from build123d import *

# Parameters (mm, degrees)
SKETCH_2_R               = 5
EXTRUDE_1_DEPTH          = 2.5
SKETCH_3_R               = 2.1
CUT_EXTRUDE_1_DEPTH      = 2.5
EXTRUDE_2_DEPTH          = 2.5
SKETCH_5_R               = 2.1
CUT_EXTRUDE_2_DEPTH      = 10
CUT_EXTRUDE_3_DEPTH      = 10
SKETCH_10_R              = 4
CUT_EXTRUDE_5_DEPTH      = 1
SKETCH_11_R              = 10
SKETCH_11_R_2            = 5
CUT_EXTRUDE_6_DEPTH      = 131.938989117
PATTERN_CIRCULAR_1_COUNT = 6


with BuildPart() as part:
    # 草图2 → 凸台-拉伸1 (new body)
    with BuildSketch(Plane(origin=(0, 0, 0), x_dir=(1, 0, 0), z_dir=(0, 1, 0))):
        Polygon((-54.5, 0), (-27.25, -47.198384506), (27.25, -47.198384506), (54.5, 0), (27.25, 47.198384506), (-27.25, 47.198384506), align=None)
        with Locations(Location((0, 0, 0), (0, 0, 270))):
            Circle(SKETCH_2_R, mode=Mode.SUBTRACT)
    extrude(amount=EXTRUDE_1_DEPTH)

    # 草图3 → 切除-拉伸1 (cut)
    with BuildSketch(Plane(origin=(0, 2.5, 0), x_dir=(1, 0, 0), z_dir=(0, 1, 0))):
        with Locations(Location((-22.5, 38.97114317, 0), (0, 0, 270))):
            Circle(SKETCH_3_R)
        with Locations(Location((22.5, 38.97114317, 0), (0, 0, 270))):
            Circle(SKETCH_3_R)
        with Locations(Location((45, 0, 0), (0, 0, 270))):
            Circle(SKETCH_3_R)
        with Locations(Location((22.5, -38.97114317, 0), (0, 0, 270))):
            Circle(SKETCH_3_R)
        with Locations(Location((-22.5, -38.97114317, 0), (0, 0, 270))):
            Circle(SKETCH_3_R)
        with Locations(Location((-45, 0, 0), (0, 0, 270))):
            Circle(SKETCH_3_R)
    extrude(amount=-CUT_EXTRUDE_1_DEPTH, mode=Mode.SUBTRACT)

    # 草图4 → 凸台-拉伸2 (add)
    with BuildSketch(Plane(origin=(0, 2.5, 0), x_dir=(1, 0, 0), z_dir=(0, 1, 0))):
        Polygon((-100.688021535, 0), (-50.344010768, -87.198384506), (50.344010768, -87.198384506), (100.688021535, 0), (50.344010768, 87.198384506), (-50.344010768, 87.198384506), align=None)
        Polygon((-54.5, 0), (-27.25, -47.198384506), (27.25, -47.198384506), (54.5, 0), (27.25, 47.198384506), (-27.25, 47.198384506), align=None, mode=Mode.SUBTRACT)
    extrude(amount=-EXTRUDE_2_DEPTH)

    # 草图5 → 切除-拉伸2 (cut)
    with BuildSketch(Plane(origin=(0, 2.5, 0), x_dir=(1, 0, 0), z_dir=(0, 1, 0))):
        with Locations(Location((-39, 67.549981495, 0), (0, 0, 270))):
            Circle(SKETCH_5_R)
        with Locations(Location((39, 67.549981495, 0), (0, 0, 270))):
            Circle(SKETCH_5_R)
        with Locations(Location((78, 0, 0), (0, 0, 270))):
            Circle(SKETCH_5_R)
        with Locations(Location((39, -67.549981495, 0), (0, 0, 270))):
            Circle(SKETCH_5_R)
        with Locations(Location((-39, -67.549981495, 0), (0, 0, 270))):
            Circle(SKETCH_5_R)
        with Locations(Location((-78, 0, 0), (0, 0, 270))):
            Circle(SKETCH_5_R)
    extrude(amount=-CUT_EXTRUDE_2_DEPTH, mode=Mode.SUBTRACT)

    # 草图8 → 切除-拉伸3 (cut)
    with BuildSketch(Plane(origin=(0, 2.5, 0), x_dir=(1, 0, 0), z_dir=(0, 1, 0))):
        with BuildLine():
            ThreePointArc((-38.999999879, 87.198384506), (-34.02771086, 86.55882369), (-29.37912053, 84.681777055))
            ThreePointArc((-29.37912053, 84.681777055), (2.23e-07, 76.996854011), (29.379120918, 84.681777273))
            ThreePointArc((29.379120918, 84.681777273), (34.027711134, 86.558823762), (39, 87.198384506))
            Line((39, 87.198384506), (-38.999999879, 87.198384506))
        make_face()
        with BuildLine():
            ThreePointArc((-58.647009902, 67.78395331), (-57.948284774, 72.748274003), (-56.016016118, 77.374183058))
            Line((-56.016016118, 77.374183058), (-95.016015856, 9.824202017))
            ThreePointArc((-95.016015856, 9.824202017), (-91.975995068, 13.810550415), (-88.026129369, 16.897824439))
            ThreePointArc((-88.026129369, 16.897824439), (-66.68123126, 38.498427568), (-58.647009902, 67.78395331))
        make_face()
        with BuildLine():
            ThreePointArc((-56.016016118, 77.374183058), (-48.824201425, 84.565997693), (-38.999999879, 87.198384506))
            Line((-38.999999879, 87.198384506), (-50.344010768, 87.198384506))
            Line((-50.344010768, 87.198384506), (-56.016016118, 77.374183058))
        make_face()
        with BuildLine():
            Line((50.344010768, 87.198384506), (39, 87.198384506))
            ThreePointArc((39, 87.198384506), (48.824200892, 84.565998001), (56.016015443, 77.374184228))
            Line((56.016015443, 77.374184228), (50.344010768, 87.198384506))
        make_face()
        with BuildLine():
            ThreePointArc((-95.016016282, -9.824201279), (-97.648403011, 4.26e-07), (-95.016015856, 9.824202017))
            Line((-95.016015856, 9.824202017), (-100.688021535, 0))
            Line((-100.688021535, 0), (-95.016016282, -9.824201279))
        make_face()
        with BuildLine():
            ThreePointArc((56.016015443, 77.374184228), (57.948284693, 72.7482743), (58.64700991, 67.783952574))
            ThreePointArc((58.64700991, 67.783952574), (66.681231635, 38.498426919), (88.026130025, 16.89782405))
            ThreePointArc((88.026130025, 16.89782405), (91.975995629, 13.810549846), (95.016016274, 9.824201294))
            Line((95.016016274, 9.824201294), (56.016015443, 77.374184228))
        make_face()
        with BuildLine():
            Line((-95.016016282, -9.824201279), (-56.016017948, -77.374179889))
            ThreePointArc((-56.016017948, -77.374179889), (-57.948285332, -72.748271969), (-58.647009908, -67.783952751))
            ThreePointArc((-58.647009908, -67.783952751), (-66.681232791, -38.498424916), (-88.026134156, -16.897821598))
            ThreePointArc((-88.026134156, -16.897821598), (-91.975997324, -13.810548132), (-95.016016282, -9.824201279))
        make_face()
        with BuildLine():
            Line((100.688021535, 0), (95.016016274, 9.824201294))
            ThreePointArc((95.016016274, 9.824201294), (97.648403011, -1.459e-06), (95.016014815, -9.824203821))
            Line((95.016014815, -9.824203821), (100.688021535, 0))
        make_face()
        with BuildLine():
            ThreePointArc((95.016014815, -9.824203821), (91.975994622, -13.810550865), (88.02613007, -16.897824023))
            ThreePointArc((88.02613007, -16.897824023), (66.681231717, -38.498426777), (58.647009914, -67.783952298))
            ThreePointArc((58.647009914, -67.783952298), (57.948284908, -72.748273515), (56.016016118, -77.374183058))
            Line((56.016016118, -77.374183058), (95.016014815, -9.824203821))
        make_face()
        with BuildLine():
            ThreePointArc((-39, -87.198384506), (-48.824203062, -84.565996748), (-56.016017948, -77.374179889))
            Line((-56.016017948, -77.374179889), (-50.344010768, -87.198384506))
            Line((-50.344010768, -87.198384506), (-39, -87.198384506))
        make_face()
        with BuildLine():
            Line((-39, -87.198384506), (39.000000014, -87.198384506))
            ThreePointArc((39.000000014, -87.198384506), (34.027710452, -86.558823583), (29.379119676, -84.681776576))
            ThreePointArc((29.379119676, -84.681776576), (-7.65e-07, -76.996854011), (-29.37912101, -84.681777325))
            ThreePointArc((-29.37912101, -84.681777325), (-34.027711185, -86.558823775), (-39, -87.198384506))
        make_face()
        with BuildLine():
            Line((50.344010768, -87.198384506), (56.016016118, -77.374183058))
            ThreePointArc((56.016016118, -77.374183058), (48.824201483, -84.565997659), (39.000000014, -87.198384506))
            Line((39.000000014, -87.198384506), (50.344010768, -87.198384506))
        make_face()
    extrude(amount=-CUT_EXTRUDE_3_DEPTH, mode=Mode.SUBTRACT)

    # 草图10 → 切除-拉伸5 (cut)
    with BuildSketch(Plane(origin=(0, 2.5, 0), x_dir=(1, 0, 0), z_dir=(0, 1, 0))):
        with Locations(Location((-78, 0, 0), (0, 0, 270))):
            Circle(SKETCH_10_R)
        with Locations(Location((-39, 67.549981495, 0), (0, 0, 270))):
            Circle(SKETCH_10_R)
        with Locations(Location((39, 67.549981495, 0), (0, 0, 270))):
            Circle(SKETCH_10_R)
        with Locations(Location((78, 0, 0), (0, 0, 270))):
            Circle(SKETCH_10_R)
        with Locations(Location((39, -67.549981495, 0), (0, 0, 270))):
            Circle(SKETCH_10_R)
        with Locations(Location((-39, -67.549981495, 0), (0, 0, 270))):
            Circle(SKETCH_10_R)
    extrude(amount=-CUT_EXTRUDE_5_DEPTH, mode=Mode.SUBTRACT)

    # 草图11 → 切除-拉伸6 (cut, through all)
    with BuildSketch(Plane.XZ):
        with BuildLine():
            Line((-34.641016151, -10), (-65.262794416, -10))
            ThreePointArc((-65.262794416, -10), (-61.72726051, -11.464466094), (-60.262794416, -15))
            ThreePointArc((-60.262794416, -15), (-63.026726517, -19.472135994), (-68.262794556, -18.999999895))
            ThreePointArc((-68.262794556, -18.999999895), (-56.291651297, -32.499999912), (-50.585879884, -49.617314069))
            ThreePointArc((-50.585879884, -49.617314069), (-45.921354555, -44.028220551), (-40.621778265, -49.019237886))
            ThreePointArc((-40.621778265, -49.019237886), (-40.792149144, -50.313333152), (-41.291651287, -51.519237957))
            Line((-41.291651287, -51.519237957), (-25.980762149, -25.000000062))
            ThreePointArc((-25.980762149, -25.000000062), (-43.301270207, -24.999999969), (-34.641016151, -10))
        make_face()
        with Locations((-34.641016151, -20)):
            Circle(SKETCH_11_R)
        with Locations((-65.262794416, -15)):
            Circle(SKETCH_11_R_2)
        with Locations((-45.621778265, -49.019237886)):
            Circle(SKETCH_11_R_2)
    cut_extrude_6 = extrude(amount=-CUT_EXTRUDE_6_DEPTH, mode=Mode.SUBTRACT)

    # 阵列(圆周)1: 切除-拉伸6 ×6 about axis
    pattern_circular_1_axis = Axis((0, 0, 0), (0, 1, 0))
    for i in range(1, PATTERN_CIRCULAR_1_COUNT):
        add(cut_extrude_6.rotate(pattern_circular_1_axis, i * 360 / PATTERN_CIRCULAR_1_COUNT), mode=Mode.SUBTRACT)


solid = part.part
The model under review builds one solid part; all positions refer to its coordinate system, in mm. A direction names the side the tool comes from. Give positions to 0.01 mm unless a question says otherwise; leave off trailing zeros. Order: outer loops, then holes, each group sorted by start corner. A loop starts at its lowest first (then second) coordinate and runs counter-clockwise, first axis right, second up. Notation, with made-up numbers: M -34,75.5 L 6,75.5 A20 cw 6,105.5 Z; hole C 36.25,-0.75 d4. An arc over 180 degrees is marked long. One line per question, with ' | ' between items. Start each with the question number.
1) Clearance check with flat-ended pins moving along their axes: P1, Ø1.5, axis at x = -30.5, y = 0.5, coming from the -Z side; P2, Ø4, axis at x = -77.5, z = 1.5, coming from the +Y side; P3, Ø1.5, axis at y = 0.5, z = -55, coming from the -X side. State where each tip first meets the part, or that it passes through.
2) Consider section A-A, the plane z = 0. State how many separate pieces and enclosed holes the cut face has, then the cut area to 3 significant figures.
3) Mouldability with a two-part tool opening along X and no side actions: class faces 1 (the face through (66.47, 1.27, -38.87)), 2 (the face through (74.095, 2.007, -0.867)) as pulls with the +X half, pulls with the -X half, needs draft (parallel to the pull), parting line crosses it, or undercut.
4) Wall thickness on L1, parallel to X at y = 1.4, z = 21.5; L2, parallel to X at y = 1.45, z = -46; L3, parallel to X at y = 2.35, z = 53.5: over which ranges is each line inside the solid? List them lowest first. Write a range as from..to.
5) Consider section D-D, the plane x = -78. Give the boundary of the cut face in (y, z), then the cut area to 3 significant figures.
6) Consider section B-B, the plane x = 0. Give the boundary of the cut face in (y, z), then the cut area to 3 significant figures.
7) For faces 3 (the face through (37, 1.5, -66)), 4 (the face through (46.7, 1.2, 53.9)), list the 3-axis set-ups (+Z, -Z, +X, -X, +Y, -Y) from which the entire face can be reached by the end or side of a thin tool; tool diameter is ignored.
Found:
1) P1: stops at z = -85.61 | P2: stops at y = 1.5 | P3: stops at x = -60.36
2) separate pieces: 6 | enclosed holes: 0 | area: 414 mm²
3) face 1: pulls with the +X half | face 2: undercut
4) L1: x = -81.34..-65.22, -24.75..24.75, 65.22..81.34 | L2: x = -63.02..-51.17, -38.11..-15.01, 15.01..38.11, 51.17..63.02 | L3: x = -60.55..-47.84, -43.4..-19.34, 19.34..43.4, 47.84..60.55
5) outline: M 0,-24.36 L 2.5,-24.36 L 2.5,-4 L 1.5,-4 L 1.5,-2.1 L 0,-2.1 Z; M 0,2.1 L 1.5,2.1 L 1.5,4 L 2.5,4 L 2.5,24.36 L 0,24.36 Z | area: 108 mm²
6) outline: M 0,-77 L 2.5,-77 L 2.5,-65 L 0,-65 Z; M 0,-30 L 2.5,-30 L 2.5,-5 L 0,-5 Z; M 0,5 L 2.5,5 L 2.5,30 L 0,30 Z; M 0,65 L 2.5,65 L 2.5,77 L 0,77 Z | area: 185 mm²
7) face 3: +Y | face 4: +Y, -Y
